Read the model definition and answer for the solid it produces. Units are mm, in the model's axes. A direction names the side the tool comes from. Give positions to 0.01 mm unless a question says otherwise; leave off trailing zeros. Order: outer loops, then holes, each group sorted by start corner. A loop starts at its lowest first (then second) coordinate and runs counter-clockwise, first axis right, second up.
```python
from build123d import *

# Parameters (mm, degrees)
SKETCH_2_R             = 47
SKETCH_2_R_2           = 37
EXTRUDE_579_DEPTH      = 16
SKETCH_3_R             = 9
EXTRUDE_773_DEPTH      = 11
SKETCH_6_W             = 4
SKETCH_6_H             = 45
CUT_EXTRUDE_1_DEPTH    = 16
FILLET_1_R             = 3
EXTRUDE_1292_DEPTH     = 50
SKETCH_18_R            = 9
CUT_EXTRUDE_1513_DEPTH = 8
FILLET_3_R             = 6
EXTRUDE_1878_DEPTH     = 8


with BuildPart() as part:
    # 草圖2 → Extrude 579 (new, symmetric)
    with BuildSketch(Plane(origin=(0, 0, 0), x_dir=(0, 0, -1), z_dir=(1, 0, 0))):
        Circle(SKETCH_2_R)
        Circle(SKETCH_2_R_2, mode=Mode.SUBTRACT)
    extrude(amount=EXTRUDE_579_DEPTH, both=True)

    # 草圖3 → Extrude 773 (add, symmetric)
    with BuildSketch(Plane.XY):
        with BuildLine():
            Line((16, 37), (-16, 37))
            Line((-16, 37), (-16, 63))
            ThreePointArc((-16, 63), (0, 79), (16, 63))
            Line((16, 63), (16, 37))
        make_face()
        with Locations((0, 63)):
            Circle(SKETCH_3_R, mode=Mode.SUBTRACT)
    extrude(amount=EXTRUDE_773_DEPTH, both=True)

    # 草圖6 → 除料-伸長1 (cut, symmetric)
    with BuildSketch(Plane(origin=(0, 0, 0), x_dir=(0, 0, -1), z_dir=(1, 0, 0))):
        with Locations((0, 59.445906404)):
            Rectangle(SKETCH_6_W, SKETCH_6_H)
    extrude(amount=CUT_EXTRUDE_1_DEPTH, both=True, mode=Mode.SUBTRACT)

    # 圓角1
    fillet_1_edges = [part.edges().sort_by_distance(p)[0] for p in [
        (0, 45.694638635, -11),
        (0, 45.694638635, 11),
    ]]
    fillet(fillet_1_edges, radius=FILLET_1_R)



with BuildPart() as body_2:
    # 草圖14 → Extrude 1292 (new, symmetric)
    with BuildSketch(Plane(origin=(0, 0, 0), x_dir=(0, 0, -1), z_dir=(1, 0, 0))):
        Polygon((-94, -47), (-86, -47), (-86, 3), (-109, 3), (-109, -12), (-94, -12), align=None)
    extrude(amount=EXTRUDE_1292_DEPTH, both=True)

    # 草圖18 → Cut-Extrude 1513 (cut)
    with BuildSketch(Plane.XY.offset(94)):
        with Locations((-34, -30)):
            Circle(SKETCH_18_R)
        with Locations((34, -30)):
            Circle(SKETCH_18_R)
    extrude(amount=-CUT_EXTRUDE_1513_DEPTH, mode=Mode.SUBTRACT)

    # 圓角3
    fillet_3_edges = [body_2.edges().sort_by_distance(p)[0] for p in [
        (50, -4.5, 109),
        (-50, -4.5, 109),
        (50, -47, 90),
        (-50, -47, 90),
    ]]
    fillet(fillet_3_edges, radius=FILLET_3_R)


with BuildPart() as part_1:
    add(part.part)

    add(body_2.part)  # Extrude 1878 merges body 2
    # 草圖20 → Extrude 1878 (add, symmetric)
    with BuildSketch(Plane(origin=(0, 0, 0), x_dir=(0, 0, -1), z_dir=(1, 0, 0))):
        with BuildLine():
            Line((-109, 3), (-19.083912356, 42.951184957))
            ThreePointArc((-19.083912356, 42.951184957), (-45.976655465, -9.754340243), (0, -47))
            Line((0, -47), (-86, -47))
            Line((-86, -47), (-86, 3))
            Line((-86, 3), (-109, 3))
        make_face()
    extrude(amount=EXTRUDE_1878_DEPTH, both=True)


solid = part_1.part
```
1) For a pull along X with two mould halves and no side action, classify faces 1 (the face through (-1.951, 54.214, -6.563)), 2 (the face through (-1.951, 54.214, 6.437)), 3 (the face through (8, -18, 62)), 4 (the face through (0.112, 22.696, 64.671)) as released by +X, released by -X, zero draft, split by the parting line, or undercut.
Final values:
face 1: undercut
face 2: undercut
face 3: released by +X
face 4: zero draft
2) The part is cut by section D-D on x = -3. Determine the outline of the cut face in (y, z), and give its area (3 significant figures).
Final values:
outline: (-47, 0) arc R47 ccw to (45.12, -13.16) arc R3 cw to (48, -11) - (54.51, -11) - (54.51, -2) - (36.95, -2) arc R37 cw (long way) to (36.95, 2) - (54.51, 2) - (54.51, 11) - (48, 11) arc R3 cw to (45.12, 13.16) arc R47 ccw to (42.95, 19.08) - (3, 109) - (-12, 109) - (-12, 94) - (-47, 94) - close; (71.49, -11) - (78.72, -11) - (78.72, -2) - (71.49, -2) - close; (71.49, 2) - (78.72, 2) - (78.72, 11) - (71.49, 11) - close
area: 6,940 mm2
3) A tool of negligible diameter and unlimited length cuts with its end or side. For faces 5 (the face through (0, 53, -2)), 6 (the face through (0.2, -15.7, -44.3)), 7 (the face through (0, 53, -11)), 8 (the face through (-16, 29, 25)), from which of +Z, -Z, +X, -X, +Y, -Y can it reach the whole face along a straight path? Write none if from no direction.
Final values:
face 5: +X, -X, +Y
face 6: none
face 7: -Z, +X, -X, +Y
face 8: -Z, -X, +Y, -Y
4) The part is cut by section C-C on y = -14.5. Determine the outline of the cut face in (x, z).
Final values:
outline: (-50, 86) - (-8, 86) - (-8, 44.71) - (-16, 44.71) - (-16, 34.04) - (16, 34.04) - (16, 44.71) - (8, 44.71) - (8, 86) - (50, 86) - (50, 94) - (-50, 94) - close; (-16, -44.71) - (16, -44.71) - (16, -34.04) - (-16, -34.04) - close
5) The part is cut by section B-B on z = 5.5. Determine the outline of the cut face in (x, y), and give its area (3 significant figures).
Final values:
outline: (-16, -46.68) - (-8, -46.68) - (-8, -47) - (8, -47) - (8, -46.68) - (16, -46.68) - (16, -36.59) - (-16, -36.59) - close; (-16, 36.59) - (16, 36.59) - (16, 63) arc R16 ccw to (-16, 63) - close; hole circle Ø18 at (0, 63)
area: 1,320 mm2
6) The part is cut by section A-A on x = 34. Determine the outline of the cut face in (y, z), and give its area (3 significant figures).
Final values:
outline: (-47, 86) - (-39, 86) - (-39, 94) - (-47, 94) - close; (-21, 86) - (3, 86) - (3, 109) - (-12, 109) - (-12, 94) - (-21, 94) - close
area: 481 mm2
7) Consider L1, parallel to Y at x = 0, z = 8; L2, parallel to Z at x = -9.5, y = -14; L3, parallel to Y at x = 0, z = -6.5. Determine where each line is inside the solid, lowest interval first.
Final values:
L1: y = -47 to -36.12, 36.12 to 54, 72 to 79
L2: z = -44.87 to -34.25, 34.25 to 44.87, 86 to 94
L3: y = -46.55 to -36.42, 36.42 to 54, 72 to 79
8) Given pin 1 (2 mm diameter, centred on x = 6.5, y = 34, fed in from -Z); pin 2 (1.5 mm diameter, centred on x = -1.5, y = 38, fed in from +Z); pin 3 (9.5 mm diameter, centred on x = -5, y = 63.5, fed in from -Z), each flat-ended and moving along its own axis, determine where each tip first touches the part or whether it passes through.
Final values:
pin 1: stops at z = -33.47
pin 2: stops at z = 31.92
pin 3: stops at z = -11
